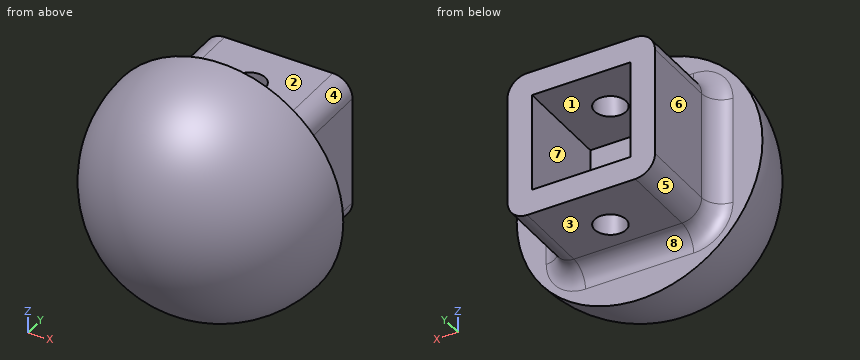
from build123d import *

# Parameters (mm, degrees)
REVOLVE2_ANGLE          = 180
SKETCH1_W               = 15
SKETCH1_H               = 15
SKETCH1_W_2             = 10
SKETCH1_H_2             = 10
BOSS_EXTRUDE1_DEPTH     = 10
SKETCH2_R               = 1.6
CUT_EXTRUDE1_DEPTH      = 20
CUT_EXTRUDE1_DEPTH_BACK = 10
FILLET1_R               = 2


with BuildPart() as part:
    # Sketch4 → Revolve2 (revolve)
    with BuildSketch(Plane(origin=(0, 0, 0), x_dir=(1, 0, 0), z_dir=(0, 1, 0))):
        with BuildLine():
            Line((12.5, 0), (-12.5, 0))
            ThreePointArc((-12.5, 0), (0, -12.5), (12.5, 0))
        make_face()
    revolve(axis=Axis((-12.5, 0, 0), (1, 0, 0)), revolution_arc=REVOLVE2_ANGLE)

    # Sketch1 → Boss-Extrude1 (add)
    with BuildSketch(Plane(origin=(0, 0, 0), x_dir=(1, 0, 0), z_dir=(0, 1, 0))):
        Rectangle(SKETCH1_W, SKETCH1_H)
        Rectangle(SKETCH1_W_2, SKETCH1_H_2, mode=Mode.SUBTRACT)
    extrude(amount=BOSS_EXTRUDE1_DEPTH)

    # Sketch2 → Cut-Extrude1 (cut, two sides)
    with BuildSketch(Plane(origin=(0, 0, 5), x_dir=(-1, 0, 0), z_dir=(0, 0, -1))) as cut_extrude1_sk:
        with Locations((0, 5)):
            Circle(SKETCH2_R)
    extrude(amount=CUT_EXTRUDE1_DEPTH, mode=Mode.SUBTRACT)
    extrude(cut_extrude1_sk.sketch, amount=-CUT_EXTRUDE1_DEPTH_BACK, mode=Mode.SUBTRACT)

    # Fillet1
    fillet1_edges = [part.edges().sort_by_distance(p)[0] for p in [
        (7.5, 0, 0),
        (7.5, 5, 7.5),
        (0, 0, -7.5),
        (7.5, 5, -7.5),
        (-7.5, 0, 0),
        (-7.5, 5, -7.5),
        (0, 0, 7.5),
        (-7.5, 5, 7.5),
    ]]
    fillet(fillet1_edges, radius=FILLET1_R)


solid = part.part
Work out the finished part from the listing and answer in its coordinate system (mm). Face numbers are marked on the shaded views. A direction names the side the tool comes from. Round coordinates to 2 decimals unless told otherwise and drop trailing zeros. Write each loop counter-clockwise with the first axis right and the second up, starting at its lowest first coordinate (ties: lowest second). Pieces come first, ordered by that corner, then holes. Notation, with made-up numbers: (-3, 55) -> (31, 55) arc R17 cw to (31, 66) -> close; hole circle Ø2 at (-29.5, 38). An arc over 180 degrees is marked (long way). Answer as CSV lines item,"result". Start each with the question number.
(1) The part is cut by section A-A, the plane x = 0. Give the vertices of the cut face in (y, z).
(2) Find the intervals of material crossed by probe 1 along Z at (x, y) = (3, 2.75); probe 2 along Y at (x, z) = (0, 5.6); probe 3 along Y at (x, z) = (0.25, 5.25), in increasing order.
(3) The part is cut by section D-D, the plane y = -10. Give the vertices of the cut face in (x, z), then the cut area to 3 significant figures.
(4) A tool of negligible diameter and unlimited length cuts with its end or side. For the marked faces 1, 2, 3, 4 and 5, from which of +Z, -Z, +X, -X, +Y, -Y can it reach the whole face along a straight path? Write none if from no direction.
(5) The mould has two halves that part along Z. Classify the marked faces 6, 7 and 8: +Z half, -Z half, draft (parallel to the pull), parting line (faces both ways), or undercut.
(6) Each of these flat-tipped pins is pushed along its axis until it touches: pin 1 (12 mm diameter, centred on y = 3.5, z = 5.5, fed in from +X); pin 2 (12 mm diameter, centred on y = -8.5, z = 9, fed in from -X); pin 3 (2 mm diameter, centred on y = 4, z = 6.5, fed in from +X). Where does it stop, or does it pass through?
(7) The part is cut by section C-C, the plane z = -2.75. Give the vertices of the cut face in (x, y), then the cut area to 3 significant figures.
(8) The part is cut by section B-B, the plane y = 5. Give the vertices of the cut face in (x, z).
Output values:
1,outline,"(0, -12.5) -> (0, -9.5) arc R2 cw to (2, -7.5) -> (3.4, -7.5) -> (3.4, -5) -> (0, -5) -> (0, 5) -> (3.4, 5) -> (3.4, 7.5) -> (2, 7.5) arc R2 cw to (0, 9.5) -> (0, 12.5) arc R12.5 ccw to start; (6.6, -7.5) -> (10, -7.5) -> (10, -5) -> (6.6, -5) -> close; (6.6, 5) -> (10, 5) -> (10, 7.5) -> (6.6, 7.5) -> close"
2,probe 1,"z = -7.5 to -5, 5 to 7.5"
2,probe 2,"y = -11.18 to 3.4, 6.6 to 10"
2,probe 3,"y = -11.34 to 3.42, 6.58 to 10"
3,outline,"circle Ø15 at (0, 0)"
3,area,"177 mm²"
4,face 1,"+Y"
4,face 2,"+Z, +X, -X, +Y"
4,face 3,"-Z, +X, -X, +Y"
4,face 4,"+Z, +X, +Y"
4,face 5,"-Z, -X, +Y"
5,face 6,"draft"
5,face 7,"undercut"
5,face 8,"-Z half"
6,pin 1,"stops at x = 12.48"
6,pin 2,"stops at x = -10.75"
6,pin 3,"stops at x = 7.5"
7,outline,"(-12.19, 0) arc R12.19 ccw to (12.19, 0) -> (9.5, 0) arc R2 cw to (7.5, 2) -> (7.5, 10) -> (5, 10) -> (5, 0) -> (-5, 0) -> (-5, 10) -> (-7.5, 10) -> (-7.5, 2) arc R2 cw to (-9.5, 0) -> close"
7,area,"285 mm²"
8,outline,"(-7.5, -5.5) arc R2 ccw to (-5.5, -7.5) -> (-1.6, -7.5) -> (-1.6, -5) -> (-5, -5) -> (-5, 5) -> (-1.6, 5) -> (-1.6, 7.5) -> (-5.5, 7.5) arc R2 ccw to (-7.5, 5.5) -> close; (1.6, -7.5) -> (5.5, -7.5) arc R2 ccw to (7.5, -5.5) -> (7.5, 5.5) arc R2 ccw to (5.5, 7.5) -> (1.6, 7.5) -> (1.6, 5) -> (5, 5) -> (5, -5) -> (1.6, -5) -> close"
